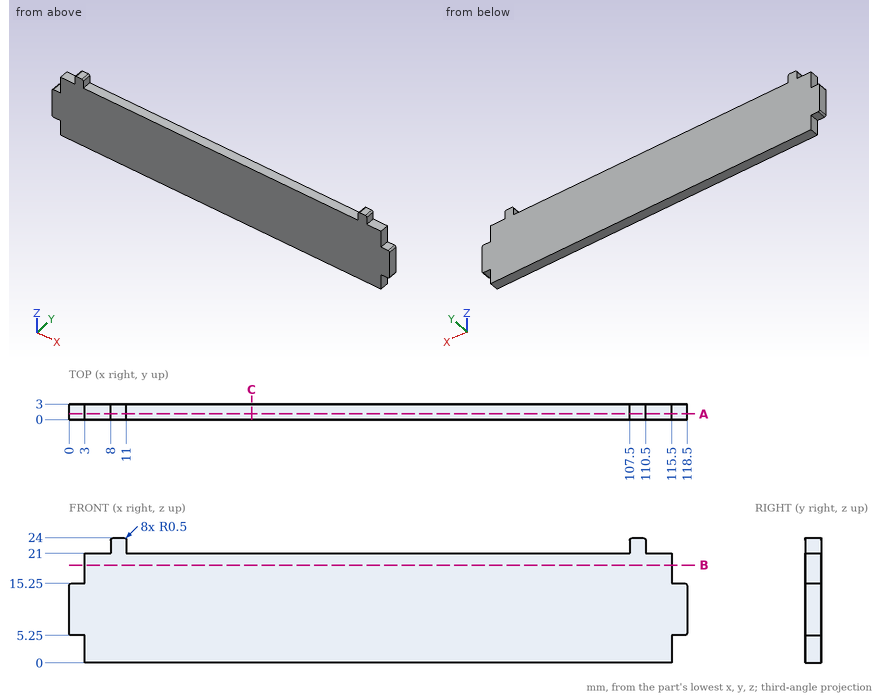
Geometry check sheet. Reference: drawing and pictorial views, mm from the part's lowest x, y, z. Coordinates: 2 decimals unless noted, no trailing zeros. Order: outer loops, then holes, each group sorted by start corner. A loop starts at its lowest first (then second) coordinate and runs counter-clockwise, first axis right, second up. Notation, with made-up numbers: (38.5, 56.5) - (73.5, 56.5) arc R34 cw to (73.5, 93.5) - close; hole circle Ø9 at (74.25, 27). An arc over 180 degrees is marked (long way). One line per item, written item: value.
(1) Thickness scan on probe 1 along Z at (x, y) = (34, 2); probe 2 along X at (y, z) = (2.6, 22.5); probe 3 along X at (y, z) = (1.4, 18.25). Record the ranges inside material, lowest first. Write a range as from..to.
Data:
probe 1: z = 0..21
probe 2: x = 8..11, 107.5..110.5
probe 3: x = 3..115.5
(2) Sectioned sample at A-A (y = 1.1). Enter the section's corners in (x, z).
Data:
outline: (0, 5.75) arc R0.5 ccw to (0.5, 5.25) - (3, 5.25) - (3, 0) - (115.5, 0) - (115.5, 5.25) - (118, 5.25) arc R0.5 ccw to (118.5, 5.75) - (118.5, 14.75) arc R0.5 ccw to (118, 15.25) - (115.5, 15.25) - (115.5, 21) - (110.5, 21) - (110.5, 23.5) arc R0.5 ccw to (110, 24) - (108, 24) arc R0.5 ccw to (107.5, 23.5) - (107.5, 21) - (11, 21) - (11, 23.5) arc R0.5 ccw to (10.5, 24) - (8.5, 24) arc R0.5 ccw to (8, 23.5) - (8, 21) - (3, 21) - (3, 15.25) - (0.5, 15.25) arc R0.5 ccw to (0, 14.75) - close
(3) Sectioned sample at B-B (z = 18.75). Enter the section's corners in (x, y).
Data:
outline: (3, 0) - (115.5, 0) - (115.5, 3) - (3, 3) - close
(4) Sectioned sample at C-C (x = 35). Enter the section's corners in (y, z), and give its area (3 significant figures).
Data:
outline: (0, 0) - (3, 0) - (3, 21) - (0, 21) - close
area: 63.0 mm^2
(5) Depth check by flat-ended pin: pin 1 Ø0.8 at (x, y) = (2, 2) entering from +Z; pin 2 Ø1.2 at (y, z) = (2, 22) entering from +X; pin 3 Ø1.5 at (y, z) = (2.5, 21) entering from +X. Enter the tip coordinate at first touch or a pass-through.
Data:
pin 1: stops at z = 15.25
pin 2: stops at x = 110.5
pin 3: stops at x = 115.5
